The listing builds one solid part. Answer for the finished solid, in the listing's coordinates (mm). Give positions to 0.01 mm unless a question says otherwise; leave off trailing zeros. Write each loop counter-clockwise with the first axis right and the second up, starting at its lowest first coordinate (ties: lowest second). Pieces come first, ordered by that corner, then holes. Notation, with made-up numbers: (53.5, 13.5) - (59.5, 13.5) arc R26 cw to (59.5, 47.5) - close; hole circle Ø3 at (76.5, -22). An arc over 180 degrees is marked (long way). Write each question's results on one line, items separated by ' | '. Start each with the question number.
Q1. Section B-B (x = -5) is taken. Determine the outline of the cut face in (y, z).
Q2. Find the intervals of material crossed by probe 1 along Y at (x, z) = (9, 1.95); probe 2 along X at (y, z) = (24.5, 1.2); probe 3 along X at (y, z) = (26, 0.25), in increasing order.
Q3. Section A-A (y = 15.5) is taken. Determine the outline of the cut face in (x, z), plus the area to 3 significant figures.
Q4. Section D-D (z = 1.5) is taken. Determine the outline of the cut face in (x, y), plus the area to 3 significant figures.
Q5. Section C-C (y = 5) is taken. Determine the outline of the cut face in (x, z), plus the area to 3 significant figures.
Q6. Flat-ended cylindrical pins translate along their axes: pin 1 Ø3 at (x, y) = (13.5, 26) entering from +Z; pin 2 Ø1 at (y, z) = (15.5, 1) entering from +X; pin 3 Ø1 at (x, z) = (14, 2) entering from +Y. Find the tip coordinate at first contact, or state that the pin passes through.
Autodesk Inventor part; units mm, degrees
ref_plane "YZ Plane" through (0, 0, 0) normal (1, 0, 0) x (0, 1, 0)
ref_plane "XZ Plane" through (0, 0, 0) normal (0, 1, 0) x (-1, 0, 0)
ref_plane "XY Plane" through (0, 0, 0) normal (0, 0, 1) x (1, 0, 0)
sketch "スケッチ1" plane through (0, 0, 0) normal (0, 0, 1) x (1, 0, 0)
  circle A0 centre (0, 15.5) radius 1.5 construction
  circle A1 centre (-13.5, 26) radius 1.25 construction
  circle A2 centre (13.5, 26) radius 1.25 construction
  circle A3 centre (-13.5, 5) radius 1.25 construction
  circle A4 centre (13.5, 5) radius 1.25 construction
  arc A5 (23.2244, 60.3803) -> (0.9204, 69.5092) centre (12.061, 64.9168) ccw
  line L0 (0.9204, 69.5092) -> (-16.5047, 27.2386)
  arc A6 (23.2244, 60.3803) -> (16.75, 27.25) centre (104.7526, 27.25) ccw
  arc A7 (-16.5047, 27.2386) -> (-16.75, 26) centre (-13.5, 26) ccw
  circle A8 centre (0, 15.5) radius 13.25
  line L1 (-16.75, 26) -> (-16.75, 3)
  line L2 (-15.75, 2) -> (-11.4155, 2)
  line L3 (11.4155, 2) -> (15.75, 2)
  arc A9 (-10.2294, 1.6104) -> (10.2294, 1.6104) centre (0, 15.5) ccw
  line L4 (16.75, 27.25) -> (16.75, 3)
  line L5 (15.75, 2) -> (16.75, 3)
  line L6 (-15.75, 2) -> (-16.75, 3)
  arc A10 (-10.2294, 1.6104) -> (-11.4155, 2) centre (-11.4155, 0) ccw
  arc A11 (11.4155, 2) -> (10.2294, 1.6104) centre (11.4155, 0) ccw
  circle A12 centre (12.061, 64.9168) radius 5 construction
  line L7 (0, 15.5) -> (0, 44.2694) construction
  point P0 (0, 0)
  point P1 (-10.7384, 2)
  point P2 (10.7384, 2)
  point P3 (16.75, 2)
  point P4 (-16.75, 2)
  dimension "d0" = 26.5
  dimension "d1" = 4
  dimension "d2" = 3
  dimension "d3" = 1
  dimension "d4" = 1
  dimension "d5" = 1
  dimension "d6" = 1
  dimension "d7" = 2
  dimension "d27" = 12.05
extrude "押し出し1" add sketch "スケッチ1" along normal blind 2
hole "穴1" at (12.061, 64.9168, 0) direction (0, 0, 1) diameter 10 end through all counterbore diameter 11.3 counterbore depth 0.65
sketch "スケッチ2" plane through (0, 0, 2) normal (0, 0, 1) x (1, 0, 0)
  circle A0 centre (13.5, 5) radius 1.25 construction
  circle A1 centre (-13.5, 5) radius 1.25 construction
  circle A2 centre (-13.5, 26) radius 1.25 construction
  circle A3 centre (13.5, 26) radius 1.25 construction
  point P0 (0, 0)
hole "穴2" at (-13.5, 5, 2) at (-13.5, 26, 2) at (13.5, 26, 2) at (13.5, 5, 2) direction (0, 0, -1) diameter 2.5 end through all countersink diameter 5.4 countersink angle 90
properties part number "UPPER_LEG_MIDDLE_FRAME_3"
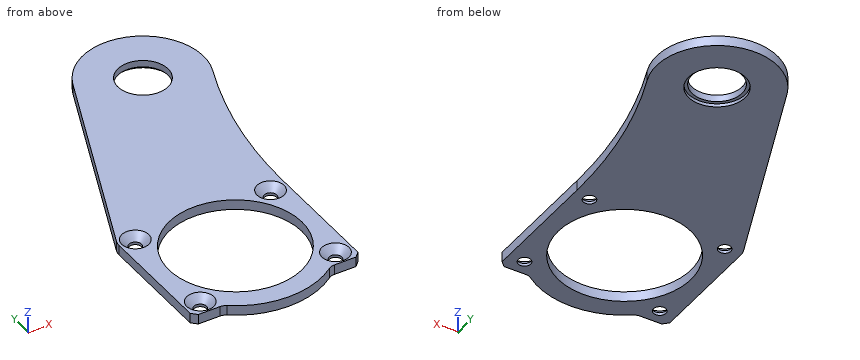
Answers below:
1) outline: (-1.01, 0) - (3.23, 0) - (3.23, 2) - (-1.01, 2) - close; (27.77, 0) - (55.15, 0) - (55.15, 2) - (27.77, 2) - close
2) probe 1: y = 0.78 to 5.78, 25.22 to 60.96, 68.87 to 76.57 | probe 2: x = -16.75 to -14.67, -12.33 to -9.72, 9.72 to 12.33, 14.67 to 16.75 | probe 3: x = -16.75 to -14.75, -12.25 to -8.08, 8.08 to 12.25, 14.75 to 16.75
3) outline: (-16.75, 0) - (-13.25, 0) - (-13.25, 2) - (-16.75, 2) - close; (13.25, 0) - (16.75, 0) - (16.75, 2) - (13.25, 2) - close | area: 14.0 mm2
4) outline: (-16.75, 3) - (-15.75, 2) - (-11.42, 2) arc R2 cw to (-10.23, 1.61) arc R17.25 ccw to (10.23, 1.61) arc R2 cw to (11.42, 2) - (15.75, 2) - (16.75, 3) - (16.75, 27.25) arc R88 cw to (23.22, 60.38) arc R12.05 ccw to (0.92, 69.51) - (-16.5, 27.24) arc R3.25 ccw to (-16.75, 26) - close; hole circle Ø4.4 at (-13.5, 5); hole circle Ø4.4 at (-13.5, 26); hole circle Ø26.5 at (0, 15.5); hole circle Ø10 at (12.06, 64.92); hole circle Ø4.4 at (13.5, 5); hole circle Ø4.4 at (13.5, 26) | area: 1,500 mm2
5) outline: (-16.75, 0) - (-14.75, 0) - (-14.75, 0.55) - (-16.2, 2) - (-16.75, 2) - close; (-12.25, 0) - (-8.08, 0) - (-8.08, 2) - (-10.8, 2) - (-12.25, 0.55) - close; (8.08, 0) - (12.25, 0) - (12.25, 0.55) - (10.8, 2) - (8.08, 2) - close; (14.75, 0) - (16.75, 0) - (16.75, 2) - (16.2, 2) - (14.75, 0.55) - close | area: 20.5 mm2
6) pin 1: stops at z = 0.8 | pin 2: stops at x = 16.75 | pin 3: stops at y = 76.88
